```python
from build123d import *

# Parameters (mm, degrees)
BOSS_EXTRUDE1_DEPTH   = 7.62
BOSS_EXTRUDE1_2_DEPTH = 7.62
BOSS_EXTRUDE1_3_DEPTH = 7.62
BOSS_EXTRUDE1_4_DEPTH = 7.62
SKETCH2_W             = 82.1538108
SKETCH2_H             = 20
BOSS_EXTRUDE2_DEPTH   = 6.35
CUT_EXTRUDE1_DEPTH    = 75.17097352
FILLET1_R             = 2.54
SKETCH13_R            = 3.5
CUT_EXTRUDE5_DEPTH    = 74.240950383
FILLET6_R             = 2.54
SKETCH14_W            = 8.89
SKETCH14_H            = 5.842
CUT_EXTRUDE6_DEPTH    = 75.17097352
SKETCH15_W            = 25.4
SKETCH15_H            = 40.894
BOSS_EXTRUDE3_DEPTH   = 12.7
FILLET15_R            = 10.16
FILLET16_R            = 10.16
FILLET17_R            = 10.16
FILLET18_R            = 10.16
SKETCH18_R            = 1.984375
CUT_EXTRUDE9_DEPTH    = 12.7


with BuildPart() as part:
    # Sketch1 → Boss-Extrude1 (new body)
    with BuildSketch(Plane(origin=(0, 0, 0), x_dir=(1, 0, 0), z_dir=(0, 1, 0))):
        Polygon((2.9718, 10), (-2.9718, 10), (-2.9718, 7.714), (-4.567901235, 7.714), (-4.567901235, 6.444), (-2.9718, 4.158), (2.9718, 4.158), (4.322098765, 6.444), (4.322098765, 7.714), (2.9718, 7.714), align=None)
    extrude(amount=BOSS_EXTRUDE1_DEPTH)



with BuildPart() as body_2:
    # Sketch1 → Boss-Extrude1 2 (new body)
    with BuildSketch(Plane(origin=(0, 0, 0), x_dir=(1, 0, 0), z_dir=(0, 1, 0))):
        Polygon((4.158, -2.9718), (4.158, 2.9718), (6.444, 4.322098765), (7.714, 4.322098765), (7.714, 2.9718), (10, 2.9718), (10, -2.9718), (7.714, -2.9718), (7.714, -4.567901235), (6.444, -4.567901235), align=None)
    extrude(amount=BOSS_EXTRUDE1_2_DEPTH)


with BuildPart() as body_3:
    # Sketch1 → Boss-Extrude1 3 (new body)
    with BuildSketch(Plane(origin=(0, 0, 0), x_dir=(1, 0, 0), z_dir=(0, 1, 0))):
        Polygon((-10, -2.9718), (-10, 2.9718), (-7.714, 2.9718), (-7.714, 4.567901235), (-6.444, 4.567901235), (-4.158, 2.9718), (-4.158, -2.9718), (-6.444, -4.322098765), (-7.714, -4.322098765), (-7.714, -2.9718), align=None)
    extrude(amount=BOSS_EXTRUDE1_3_DEPTH)


with BuildPart() as body_4:
    # Sketch1 → Boss-Extrude1 4 (new body)
    with BuildSketch(Plane(origin=(0, 0, 0), x_dir=(1, 0, 0), z_dir=(0, 1, 0))):
        Polygon((4.567901235, -6.444), (2.9718, -4.158), (-2.9718, -4.158), (-4.322098765, -6.444), (-4.322098765, -7.714), (-2.9718, -7.714), (-2.9718, -10), (2.9718, -10), (2.9718, -7.714), (4.567901235, -7.714), align=None)
    extrude(amount=BOSS_EXTRUDE1_4_DEPTH)


with BuildPart() as part_1:
    add(part.part)

    add(body_2.part)  # Boss-Extrude2 merges body 2

    add(body_3.part)  # Boss-Extrude2 merges body 3

    add(body_4.part)  # Boss-Extrude2 merges body 4
    # Sketch2 → Boss-Extrude2 (add)
    with BuildSketch(Plane.XZ):
        with Locations((-31.0769054, 0)):
            Rectangle(SKETCH2_W, SKETCH2_H)
    extrude(amount=BOSS_EXTRUDE2_DEPTH)

    # Sketch4 → Cut-Extrude1 (cut, through all)
    with BuildSketch(Plane(origin=(0, -6.35, 0), x_dir=(-1, 0, 0), z_dir=(0, -1, 0))):
        Polygon((72.1538108, -10), (34.6126108, -10), (72.1538108, -0.2108), align=None)
    extrude(amount=-CUT_EXTRUDE1_DEPTH, mode=Mode.SUBTRACT)

    # Fillet1
    fillet1_edges = [part_1.edges().sort_by_distance(p)[0] for p in [
        (-34.6126108, -3.175, 10),
    ]]
    fillet(fillet1_edges, radius=FILLET1_R)

    # Sketch13 → Cut-Extrude5 (cut, through all)
    with BuildSketch(Plane(origin=(0, 0, 0), x_dir=(1, 0, 0), z_dir=(0, 1, 0))):
        with Locations(Location((0, 0, 0), (0, 0, 270))):
            Circle(SKETCH13_R)
    extrude(amount=-CUT_EXTRUDE5_DEPTH, mode=Mode.SUBTRACT)

    # Fillet6
    fillet6_edges = [part_1.edges().sort_by_distance(p)[0] for p in [
        (0, -6.35, -3.5),
    ]]
    fillet(fillet6_edges, radius=FILLET6_R)

    # Sketch14 → Cut-Extrude6 (cut, through all)
    with BuildSketch(Plane(origin=(0, 7.62, 0), x_dir=(1, 0, 0), z_dir=(0, 1, 0))):
        with Locations((-0.122901235, 7.079)):
            Rectangle(SKETCH14_W, SKETCH14_H)
    extrude(amount=-CUT_EXTRUDE6_DEPTH, mode=Mode.SUBTRACT)

    # Sketch15 → Boss-Extrude3 (add)
    with BuildSketch(Plane.ZY.offset(72.1538108)):
        with Locations((-12.4892, -20.447)):
            Rectangle(SKETCH15_W, SKETCH15_H)
    extrude(amount=-BOSS_EXTRUDE3_DEPTH)

    # Fillet15
    fillet15_edges = [part_1.edges().sort_by_distance(p)[0] for p in [
        (-59.4538108, -6.35, -4.8946),
    ]]
    fillet(fillet15_edges, radius=FILLET15_R)

    # Fillet16
    fillet16_edges = [part_1.edges().sort_by_distance(p)[0] for p in [
        (-59.4538108, -8.255, -10),
    ]]
    fillet(fillet16_edges, radius=FILLET16_R)

    # Fillet17
    fillet17_edges = [part_1.edges().sort_by_distance(p)[0] for p in [
        (-59.4538108, -40.894, -12.4892),
    ]]
    fillet(fillet17_edges, radius=FILLET17_R)

    # Fillet18
    fillet18_edges = [part_1.edges().sort_by_distance(p)[0] for p in [
        (-56.478015697, -9.325795103, 0.2108),
        (-70.8838108, -40.894, 0.2108),
        (-59.4538108, -23.622, 0.2108),
        (-62.429605903, -37.918204897, 0.2108),
    ]]
    fillet(fillet18_edges, radius=FILLET18_R)

    # Sketch18 → Cut-Extrude9 (cut)
    with BuildSketch(Plane.ZY.offset(72.1538108)):
        with Locations((-12.4892, -28.194)):
            Circle(SKETCH18_R)
    extrude(amount=-CUT_EXTRUDE9_DEPTH, mode=Mode.SUBTRACT)


solid = part_1.part
```
CAD build for the part. Positions are in the model's coordinates, mm. A direction names the side the tool comes from. Give positions to 0.01 mm unless a question says otherwise; leave off trailing zeros. Order: outer loops, then holes, each group sorted by start corner. A loop starts at its lowest first (then second) coordinate and runs counter-clockwise, first axis right, second up. Notation, with made-up numbers: M -29,38.5 L 30,38.5 A26 cw 30,53.5 Z; hole C -6.75,55.5 d6. An arc over 180 degrees is marked long. Put each result on its own line as item: value. Start each with the question number.
(1) Flat gauge pins, fed straight in: pin 1 Ø0.7 at (y, z) = (2.5, 9) entering from +X; pin 2 Ø1.3 at (y, z) = (5, -4) entering from -X; pin 3 Ø1.9 at (x, y) = (-28, -2) entering from -Z; pin 4 Ø5.5 at (x, z) = (0, 0) entering from -Y. Where does each tip first touch, or does it go through?
(2) Which spindle directions (+Z, -Z, +X, -X, +Y, -Y) get a long thin tool onto all of the face, cutting with end or side? Do faces 1 (the flat face through (4.158, 4, 0)), 2 (the flat face through (0, -3, -4.158)), 3 (the cylindrical face through (-62.509, -23.522, -2.686)). Say none if no direction does.
(3) Saw through at C-C, the plane x = 0. Write the cut outline in (y, z).
(4) Saw through at B-B, the plane z = -13. Write the cut outline in (x, y).
(5) Saw through at A-A, the plane y = -1. Write the cut outline in (x, z), then the cut area to 3 significant figures.
(6) Saw through at D-D, the plane y = -36. Write the cut outline in (x, z), then the cut area to 3 significant figures.
(7) Drill centre lines: line 1 along Y through (x, z) = (-26, 4.5); line 2 along X through (y, z) = (-1, 0); line 3 along X through (y, z) = (-35, -23). Where is each one in solid material? Low to high.
(8) Mould opens along X. For faces 4 (the flat face through (4, 4, 7.714)), 5 (the flat face through (0, 4, 4.158)), 6 (the flat face through (2.972, 4, 9)) say: +X half, -X half, draft (parallel to the pull), parting line (faces both ways), or undercut.
Check result:
1. pin 1: stops at x = 2.97
1. pin 2: stops at x = -7.71
1. pin 3: stops at z = -10
1. pin 4: passes through
2. face 1: -Z, +Y
2. face 2: -Z, +Y, -Y
2. face 3: +Z, +X, -Y
3. outline: M -6.35,6.04 A2.54 ccw -3.81,3.5 L 0,3.5 L 0,4.16 L 7.62,4.16 L 7.62,10 L -6.35,10 Z; M -5.52,-4.16 L 0,-4.16 L 0,-3.5 L -3.81,-3.5 A2.54 ccw Z
4. outline: M -72.15,-40.89 L -69.61,-40.89 A10.16 ccw -59.45,-30.73 L -59.45,-30.11 L -72.15,-30.11 Z; M -72.15,-26.28 L -59.45,-26.28 L -59.45,-16.51 A10.16 cw -56.5,-9.35 L -56.5,0 L -72.15,0 Z
5. outline: M -72.15,-25.19 L -59.45,-25.19 L -59.45,-20.16 A10.16 cw -49.29,-10 L -4.57,-10 L -4.57,-4.16 L 4.32,-4.16 L 4.32,-10 L 10,-10 L 10,10 L -34.29,10 A2.54 ccw -34.93,9.92 L -72.15,0.21 Z; hole C 0,0 d7
5. area: 1,580 mm2
6. outline: M -72.15,-25.19 L -60.93,-25.19 L -60.93,-9.95 A8.69 ccw -69.61,-1.26 L -72.15,-1.26 Z
6. area: 252 mm2
7. line 1: y = -6.35 to 0
7. line 2: x = -72.15 to -3.5, 3.5 to 10
7. line 3: x = -72.15 to -60.39
8. face 4: draft
8. face 5: undercut
8. face 6: +X half
